```python
from build123d import *

# Parameters (mm, degrees)
SKETCH1_R           = 1.355900406
BOSS_EXTRUDE1_DEPTH = 1.5875
SKETCH2_R           = 3.175
BOSS_EXTRUDE2_DEPTH = 1.5875


with BuildPart() as part:
    # Sketch1 → Boss-Extrude1 (new body)
    with BuildSketch(Plane.XY):
        with BuildLine():
            Line((-301.9473, 111.74645), (-305.87795, 115.6771))
            Line((-305.87795, 115.6771), (-316.1078, 115.6771))
            Line((-316.1078, 115.6771), (-316.1078, 128.8851))
            Line((-316.1078, 128.8851), (-305.87795, 128.8851))
            Line((-305.87795, 128.8851), (-301.9473, 132.81575))
            Line((-301.9473, 132.81575), (-301.9473, 150.9704))
            ThreePointArc((-301.9473, 150.9704), (-303.063223164, 153.664476836), (-305.7573, 154.7804))
            Line((-305.7573, 154.7804), (-397.247125, 154.7804))
            ThreePointArc((-397.247125, 154.7804), (-399.946077222, 153.659592612), (-401.0571, 150.956597849))
            Line((-401.0571, 150.956597849), (-401.0571, 148.341))
            Line((-401.0571, 148.341), (-399.1521, 148.341))
            Line((-399.1521, 148.341), (-399.1521, 95.6449))
            Line((-399.1521, 95.6449), (-401.0571, 95.6449))
            Line((-401.0571, 95.6449), (-401.0571, 91.659304166))
            ThreePointArc((-401.0571, 91.659304166), (-399.951018769, 88.947400452), (-397.2472, 87.8217))
            Line((-397.2472, 87.8217), (-378.5565, 87.8217))
            Line((-378.5565, 87.8217), (-368.3165, 91.1883))
            Line((-368.3165, 91.1883), (-315.9973, 91.1883))
            Line((-315.9973, 91.1883), (-305.7573, 87.8217))
            ThreePointArc((-305.7573, 87.8217), (-303.063223164, 88.937623164), (-301.9473, 91.6317))
            Line((-301.9473, 91.6317), (-301.9473, 111.74645))
        make_face()
        with Locations((-305.7573, 91.6317)):
            Circle(SKETCH1_R, mode=Mode.SUBTRACT)
        with Locations((-305.7573, 150.9704)):
            Circle(SKETCH1_R, mode=Mode.SUBTRACT)
        with Locations((-397.247125, 150.9704)):
            Circle(SKETCH1_R, mode=Mode.SUBTRACT)
        with Locations((-397.2472, 91.6317)):
            Circle(SKETCH1_R, mode=Mode.SUBTRACT)
    extrude(amount=BOSS_EXTRUDE1_DEPTH)

    # Sketch2 → Boss-Extrude2 (add)
    # profile 1 of 2: a face of its own
    with BuildSketch(Plane.XY.offset(1.5875)):
        with BuildLine():
            Line((-361.0272, 165.75105), (-361.0272, 154.7804))
            Line((-361.0272, 154.7804), (-341.9772, 154.7804))
            Line((-341.9772, 154.7804), (-341.9772, 165.75105))
            ThreePointArc((-341.9772, 165.75105), (-351.5022, 175.27605), (-361.0272, 165.75105))
        make_face()
        with Locations((-351.5022, 165.75105)):
            Circle(SKETCH2_R, mode=Mode.SUBTRACT)
    # profile 2 of 2: a face of its own
    with BuildSketch(Plane.XY.offset(1.5875)):
        with BuildLine():
            Line((-341.9772, 91.1883), (-361.0272, 91.1883))
            Line((-361.0272, 91.1883), (-361.0272, 76.85105))
            ThreePointArc((-361.0272, 76.85105), (-351.5022, 67.32605), (-341.9772, 76.85105))
            Line((-341.9772, 76.85105), (-341.9772, 91.1883))
        make_face()
        with Locations((-351.5022, 76.85105)):
            Circle(SKETCH2_R, mode=Mode.SUBTRACT)
    extrude(amount=-BOSS_EXTRUDE2_DEPTH)


solid = part.part
```
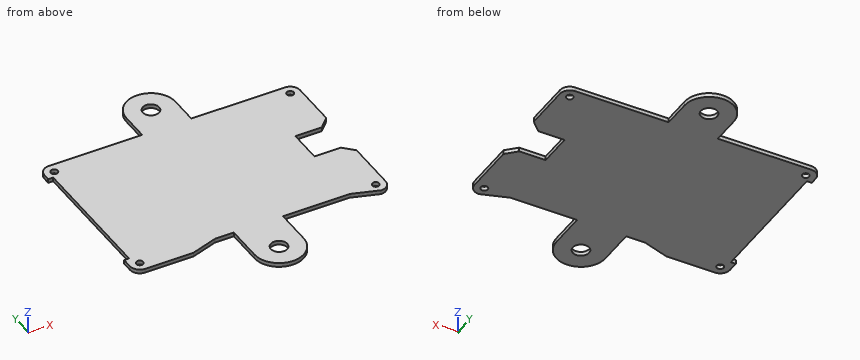
Input: part model. Units: mm. Frame: model coordinates. Coordinates: 2 decimals unless noted, no trailing zeros. Write each loop counter-clockwise with the first axis right and the second up, starting at its lowest first coordinate (ties: lowest second). Pieces come first, ordered by that corner, then holes.
1) Pin query (flat end, axial travel): pin 1 Ø0.8 at (x, z) = (-392, 1) entering from -Y; pin 2 Ø2.5 at (x, y) = (-305.76, 150.97) entering from +Z; pin 3 Ø0.8 at (y, z) = (162, 0.5) entering from -X; pin 4 Ø0.5 at (x, z) = (-365.5, 1) entering from -Y. Return the tip coordinate at first contact, or that it passes through.
2) Section C-C on z = 1.25. State how many separate pieces and enclosed holes the cut face has, and give its area (3 significant figures).
3) Section A-A on x = -389.5. Output: boundary loops of the cut face in (y, z).
4) Section B-B on y = 122. Output: boundary loops of the cut face in (x, z).
5) Material intervals for line 1 along Y through (x, z) = (-379, 1.25); line 2 along X through (y, z) = (158.5, 0.1); line 3 along Y through (x, z) = (-339, 0.85), sorted ascending.
Check result:
1. pin 1: stops at y = 87.82
1. pin 2: passes through
1. pin 3: stops at x = -361.03
1. pin 4: stops at y = 91.19
2. separate pieces: 1
2. enclosed holes: 6
2. area: 6,790 mm2
3. outline: (87.82, 0) - (154.78, 0) - (154.78, 1.59) - (87.82, 1.59) - close
4. outline: (-399.15, 0) - (-316.11, 0) - (-316.11, 1.59) - (-399.15, 1.59) - close
5. line 1: y = 87.82 to 154.78
5. line 2: x = -361.03 to -341.98
5. line 3: y = 91.19 to 154.78
